Design review of the part built by this model. Coordinates are the model's own, in mm. Coordinates: 2 decimals unless noted, no trailing zeros. Loops run counter-clockwise (first coordinate to the right, second up) from the corner with the lowest first, then second, coordinate; pieces in that order, holes last. Notation, with made-up numbers: (86, 42.25) - (129, 42.25) arc R26 ccw to (129, 56.25) - close; hole circle Ø11 at (11.5, -10). An arc over 180 degrees is marked (long way). Use one line per item in the form item = value. Start each with the question number.
(1) Add section A-A (z = 964.5). State the section outline as (x, y) points.
(2) Add section B-B (x = 1036). State the section outline as (y, z) points.
(3) For L1, parallel to X at y = -10, z = 120; L2, parallel to X at y = -23, z = 812; L3, parallel to Z at x = 787.5, y = -14.5, list the stretches that pass through material, from the lowest coordinate up.
(4) Clearance check with flat-ended pins moving along their axes: pin 1 Ø4 at (y, z) = (-4, 546) entering from -X; pin 2 Ø4 at (x, z) = (907.5, 194) entering from +Y; pin 3 Ø10 at (x, z) = (768.5, 589) entering from +Y. State where each tip first meets the part, or that it passes through.
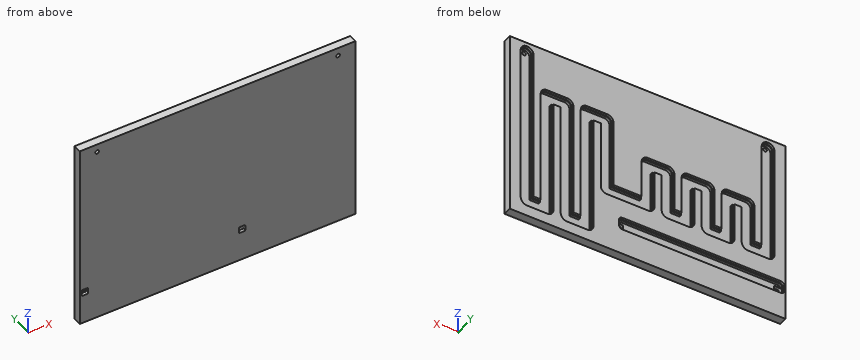
```python
from build123d import *

# Parameters (mm, degrees)
SKETCH_1_W          = 1515
SKETCH_1_H          = 1035
EXTRUDE_1_DEPTH     = 45
CUT_EXTRUDE_1_DEPTH = 13
CUT_EXTRUDE_2_DEPTH = 27
CUT_EXTRUDE_3_DEPTH = 45
CUT_EXTRUDE_5_DEPTH = 13
CUT_EXTRUDE_6_DEPTH = 27
SKETCH_3_R          = 10.25
CUT_EXTRUDE_7_DEPTH = 45


with BuildPart() as part:
    # Sketch 1 → Extrude 1 (new body)
    with BuildSketch(Plane(origin=(0, 0, 0), x_dir=(1, 0, 0), z_dir=(0, 1, 0))):
        with Locations((757.5, -517.5)):
            Rectangle(SKETCH_1_W, SKETCH_1_H)
    extrude(amount=-EXTRUDE_1_DEPTH)

    # Sketch 1_3 → Cut-Extrude 1 (cut)
    with BuildSketch(Plane(origin=(0, 0, 0), x_dir=(1, 0, 0), z_dir=(0, 1, 0))):
        with BuildLine():
            Line((5, -195), (5, -165))
            ThreePointArc((5, -165), (10.857864376, -150.857864376), (25, -145))
            Line((25, -145), (895, -145))
            ThreePointArc((895, -145), (909.142135624, -150.857864376), (915, -165))
            Line((915, -165), (915, -195))
            ThreePointArc((915, -195), (909.142135624, -209.142135624), (895, -215))
            Line((895, -215), (25, -215))
            ThreePointArc((25, -215), (10.857864376, -209.142135624), (5, -195))
        make_face()
    extrude(amount=-CUT_EXTRUDE_1_DEPTH, mode=Mode.SUBTRACT)

    # Sketch 1_5 → Cut-Extrude 2 (cut)
    with BuildSketch(Plane(origin=(0, 0, 0), x_dir=(1, 0, 0), z_dir=(0, 1, 0))):
        with BuildLine():
            Line((25, -150), (895, -150))
            ThreePointArc((895, -150), (905.606601718, -154.393398282), (910, -165))
            Line((910, -165), (910, -195))
            ThreePointArc((910, -195), (905.606601718, -205.606601718), (895, -210))
            Line((895, -210), (25, -210))
            ThreePointArc((25, -210), (14.393398282, -205.606601718), (10, -195))
            Line((10, -195), (10, -165))
            ThreePointArc((10, -165), (14.393398282, -154.393398282), (25, -150))
        make_face()
    extrude(amount=-CUT_EXTRUDE_2_DEPTH, mode=Mode.SUBTRACT)

    # Sketch 1_6 → Cut-Extrude 3 (cut)
    with BuildSketch(Plane(origin=(0, 0, 0), x_dir=(1, 0, 0), z_dir=(0, 1, 0))):
        with BuildLine():
            Line((40, -197.5), (15, -197.5))
            ThreePointArc((15, -197.5), (11.464466094, -196.035533906), (10, -192.5))
            Line((10, -192.5), (10, -167.5))
            ThreePointArc((10, -167.5), (11.464466094, -163.964466094), (15, -162.5))
            Line((15, -162.5), (40, -162.5))
            ThreePointArc((40, -162.5), (43.535533906, -163.964466094), (45, -167.5))
            Line((45, -167.5), (45, -192.5))
            ThreePointArc((45, -192.5), (43.535533906, -196.035533906), (40, -197.5))
        make_face()
        with BuildLine():
            Line((905, -197.5), (880, -197.5))
            ThreePointArc((880, -197.5), (876.464466094, -196.035533906), (875, -192.5))
            Line((875, -192.5), (875, -167.5))
            ThreePointArc((875, -167.5), (876.464466094, -163.964466094), (880, -162.5))
            Line((880, -162.5), (905, -162.5))
            ThreePointArc((905, -162.5), (908.535533906, -163.964466094), (910, -167.5))
            Line((910, -167.5), (910, -192.5))
            ThreePointArc((910, -192.5), (908.535533906, -196.035533906), (905, -197.5))
        make_face()
    extrude(amount=-CUT_EXTRUDE_3_DEPTH, mode=Mode.SUBTRACT)

    # Sketch 1_9 → Cut-Extrude 5 (cut)
    with BuildSketch(Plane(origin=(0, 0, 0), x_dir=(1, 0, 0), z_dir=(0, 1, 0))):
        with BuildLine():
            Line((60, -980), (60, -355))
            ThreePointArc((60, -355), (70.251262658, -330.251262658), (95, -320))
            Line((95, -320), (205, -320))
            ThreePointArc((205, -320), (229.748737342, -330.251262658), (240, -355))
            Line((240, -355), (240, -565))
            Line((240, -565), (280, -565))
            Line((280, -565), (280, -355))
            ThreePointArc((280, -355), (290.251262658, -330.251262658), (315, -320))
            Line((315, -320), (425, -320))
            ThreePointArc((425, -320), (449.748737342, -330.251262658), (460, -355))
            Line((460, -355), (460, -565))
            Line((460, -565), (500, -565))
            Line((500, -565), (500, -355))
            ThreePointArc((500, -355), (510.251262658, -330.251262658), (535, -320))
            Line((535, -320), (645, -320))
            ThreePointArc((645, -320), (669.748737342, -330.251262658), (680, -355))
            Line((680, -355), (680, -565))
            Line((680, -565), (720, -565))
            Line((720, -565), (720, -355))
            ThreePointArc((720, -355), (730.251262658, -330.251262658), (755, -320))
            Line((755, -320), (980, -320))
            ThreePointArc((980, -320), (1004.748737342, -330.251262658), (1015, -355))
            Line((1015, -355), (1015, -730))
            Line((1015, -730), (1055, -730))
            Line((1055, -730), (1055, -95))
            ThreePointArc((1055, -95), (1065.251262658, -70.251262658), (1090, -60))
            Line((1090, -60), (1200, -60))
            ThreePointArc((1200, -60), (1224.748737342, -70.251262658), (1235, -95))
            Line((1235, -95), (1235, -730))
            Line((1235, -730), (1275, -730))
            Line((1275, -730), (1275, -95))
            ThreePointArc((1275, -95), (1285.251262658, -70.251262658), (1310, -60))
            Line((1310, -60), (1420, -60))
            ThreePointArc((1420, -60), (1444.748737342, -70.251262658), (1455, -95))
            Line((1455, -95), (1455, -980))
            ThreePointArc((1455, -980), (1420, -1015), (1385, -980))
            Line((1385, -980), (1385, -130))
            Line((1385, -130), (1345, -130))
            Line((1345, -130), (1345, -765))
            ThreePointArc((1345, -765), (1334.748737342, -789.748737342), (1310, -800))
            Line((1310, -800), (1200, -800))
            ThreePointArc((1200, -800), (1175.251262658, -789.748737342), (1165, -765))
            Line((1165, -765), (1165, -130))
            Line((1165, -130), (1125, -130))
            Line((1125, -130), (1125, -765))
            ThreePointArc((1125, -765), (1114.748737342, -789.748737342), (1090, -800))
            Line((1090, -800), (980, -800))
            ThreePointArc((980, -800), (955.251262658, -789.748737342), (945, -765))
            Line((945, -765), (945, -390))
            Line((945, -390), (790, -390))
            Line((790, -390), (790, -600))
            ThreePointArc((790, -600), (779.748737342, -624.748737342), (755, -635))
            Line((755, -635), (645, -635))
            ThreePointArc((645, -635), (620.251262658, -624.748737342), (610, -600))
            Line((610, -600), (610, -390))
            Line((610, -390), (570, -390))
            Line((570, -390), (570, -600))
            ThreePointArc((570, -600), (559.748737342, -624.748737342), (535, -635))
            Line((535, -635), (425, -635))
            ThreePointArc((425, -635), (400.251262658, -624.748737342), (390, -600))
            Line((390, -600), (390, -390))
            Line((390, -390), (350, -390))
            Line((350, -390), (350, -600))
            ThreePointArc((350, -600), (339.748737342, -624.748737342), (315, -635))
            Line((315, -635), (205, -635))
            ThreePointArc((205, -635), (180.251262658, -624.748737342), (170, -600))
            Line((170, -600), (170, -390))
            Line((170, -390), (130, -390))
            Line((130, -390), (130, -980))
            ThreePointArc((130, -980), (95, -1015), (60, -980))
        make_face()
    extrude(amount=-CUT_EXTRUDE_5_DEPTH, mode=Mode.SUBTRACT)

    # Sketch 1_10 → Cut-Extrude 6 (cut)
    with BuildSketch(Plane(origin=(0, 0, 0), x_dir=(1, 0, 0), z_dir=(0, 1, 0))):
        with BuildLine():
            Line((1390, -980), (1390, -125))
            Line((1390, -125), (1340, -125))
            Line((1340, -125), (1340, -765))
            ThreePointArc((1340, -765), (1331.213203436, -786.213203436), (1310, -795))
            Line((1310, -795), (1200, -795))
            ThreePointArc((1200, -795), (1178.786796564, -786.213203436), (1170, -765))
            Line((1170, -765), (1170, -125))
            Line((1170, -125), (1120, -125))
            Line((1120, -125), (1120, -765))
            ThreePointArc((1120, -765), (1111.213203436, -786.213203436), (1090, -795))
            Line((1090, -795), (980, -795))
            ThreePointArc((980, -795), (958.786796564, -786.213203436), (950, -765))
            Line((950, -765), (950, -385))
            Line((950, -385), (785, -385))
            Line((785, -385), (785, -600))
            ThreePointArc((785, -600), (776.213203436, -621.213203436), (755, -630))
            Line((755, -630), (645, -630))
            ThreePointArc((645, -630), (623.786796564, -621.213203436), (615, -600))
            Line((615, -600), (615, -385))
            Line((615, -385), (565, -385))
            Line((565, -385), (565, -600))
            ThreePointArc((565, -600), (556.213203436, -621.213203436), (535, -630))
            Line((535, -630), (425, -630))
            ThreePointArc((425, -630), (403.786796564, -621.213203436), (395, -600))
            Line((395, -600), (395, -385))
            Line((395, -385), (345, -385))
            Line((345, -385), (345, -600))
            ThreePointArc((345, -600), (336.213203436, -621.213203436), (315, -630))
            Line((315, -630), (205, -630))
            ThreePointArc((205, -630), (183.786796564, -621.213203436), (175, -600))
            Line((175, -600), (175, -385))
            Line((175, -385), (125, -385))
            Line((125, -385), (125, -980))
            ThreePointArc((125, -980), (95, -1010), (65, -980))
            Line((65, -980), (65, -355))
            ThreePointArc((65, -355), (73.786796564, -333.786796564), (95, -325))
            Line((95, -325), (205, -325))
            ThreePointArc((205, -325), (226.213203436, -333.786796564), (235, -355))
            Line((235, -355), (235, -570))
            Line((235, -570), (285, -570))
            Line((285, -570), (285, -355))
            ThreePointArc((285, -355), (293.786796564, -333.786796564), (315, -325))
            Line((315, -325), (425, -325))
            ThreePointArc((425, -325), (446.213203436, -333.786796564), (455, -355))
            Line((455, -355), (455, -570))
            Line((455, -570), (505, -570))
            Line((505, -570), (505, -355))
            ThreePointArc((505, -355), (513.786796564, -333.786796564), (535, -325))
            Line((535, -325), (645, -325))
            ThreePointArc((645, -325), (666.213203436, -333.786796564), (675, -355))
            Line((675, -355), (675, -570))
            Line((675, -570), (725, -570))
            Line((725, -570), (725, -355))
            ThreePointArc((725, -355), (733.786796564, -333.786796564), (755, -325))
            Line((755, -325), (980, -325))
            ThreePointArc((980, -325), (1001.213203436, -333.786796564), (1010, -355))
            Line((1010, -355), (1010, -735))
            Line((1010, -735), (1060, -735))
            Line((1060, -735), (1060, -95))
            ThreePointArc((1060, -95), (1068.786796564, -73.786796564), (1090, -65))
            Line((1090, -65), (1200, -65))
            ThreePointArc((1200, -65), (1221.213203436, -73.786796564), (1230, -95))
            Line((1230, -95), (1230, -735))
            Line((1230, -735), (1280, -735))
            Line((1280, -735), (1280, -95))
            ThreePointArc((1280, -95), (1288.786796564, -73.786796564), (1310, -65))
            Line((1310, -65), (1420, -65))
            ThreePointArc((1420, -65), (1441.213203436, -73.786796564), (1450, -95))
            Line((1450, -95), (1450, -980))
            ThreePointArc((1450, -980), (1420, -1010), (1390, -980))
        make_face()
    extrude(amount=-CUT_EXTRUDE_6_DEPTH, mode=Mode.SUBTRACT)

    # Sketch 3 → Cut-Extrude 7 (cut)
    with BuildSketch(Plane(origin=(0, 0, 0), x_dir=(1, 0, 0), z_dir=(0, 1, 0))):
        with Locations(Location((95, -990, 0), (0, 0, 270))):
            Circle(SKETCH_3_R)
        with Locations(Location((1420, -990, 0), (0, 0, 270))):
            Circle(SKETCH_3_R)
    extrude(amount=-CUT_EXTRUDE_7_DEPTH, mode=Mode.SUBTRACT)


solid = part.part
```
Computed values:
q1.outline = (0, -45) - (1515, -45) - (1515, 0) - (1455, 0) - (1455, -13) - (1450, -13) - (1450, -27) - (1390, -27) - (1390, -13) - (1385, -13) - (1385, 0) - (130, 0) - (130, -13) - (125, -13) - (125, -27) - (65, -27) - (65, -13) - (60, -13) - (60, 0) - (0, 0) - close
q2.outline = (-45, 0) - (0, 0) - (0, 730) - (-13, 730) - (-13, 735) - (-27, 735) - (-27, 795) - (-13, 795) - (-13, 800) - (0, 800) - (0, 1035) - (-45, 1035) - close
q3.L1 = 0 to 1055, 1235 to 1275, 1455 to 1515
q3.L2 = 0 to 65, 125 to 1390, 1450 to 1515
q3.L3 = 0 to 150, 210 to 325, 385 to 1035
q4.pin_1 = 0
q4.pin_2 = through
q4.pin_3 = -27
